```python
from build123d import *

# Parameters (mm, degrees)
SKETCH_W     = 12
SKETCH_H     = 12.3
PAD_DEPTH    = 2
SKETCH001_W  = 1.8
SKETCH001_H  = 2.7
POCKET_DEPTH = 0.2
PAD001_DEPTH = 13
CHAMFER_SIZE = 1


with BuildPart() as part:
    # Sketch → Pad (new body)
    with BuildSketch(Plane.XY):
        with Locations((6, 6.15)):
            Rectangle(SKETCH_W, SKETCH_H)
    extrude(amount=PAD_DEPTH)

    # Sketch001 (on Face5 of Pad) → Pocket (cut)
    with BuildSketch(Plane(origin=(0, 0, 0), x_dir=(1, 0, 0), z_dir=(0, 0, -1))):
        with Locations((6.2, -3.25)):
            Rectangle(SKETCH001_W, SKETCH001_H)
        with Locations((6.2, -9.05)):
            Rectangle(SKETCH001_W, SKETCH001_H)
    extrude(amount=-POCKET_DEPTH, mode=Mode.SUBTRACT)

    # Sketch002 (on Face1 of Pocket) → Pad001 (join)
    with BuildSketch(Plane.XZ):
        with BuildLine():
            ThreePointArc((11.16, 0.23875), (16.969381, -4.45007), (22.238211, 0.838915))
            Line((21.467655, 1.119375), (22.238211, 0.838915))
            ThreePointArc((12, 0), (17.23124, -3.647424), (21.467655, 1.119375))
            Line((12, 2), (12, 0))
            ThreePointArc((20.026412, 4.478132), (15.266374, 5.657977), (12, 2))
            Line((20.026412, 4.478132), (20.026412, 5.572296))
            ThreePointArc((20.026412, 5.572296), (14.583244, 6.292865), (11.16, 2))
            Line((11.16, 2), (11.16, 0.23875))
        make_face()
    extrude(amount=-PAD001_DEPTH)

    # Chamfer
    chamfer_edges = [part.edges().sort_by_distance(p)[0] for p in [
        (0, 6.15, 2),
    ]]
    chamfer(chamfer_edges, length=CHAMFER_SIZE)


solid = part.part
```
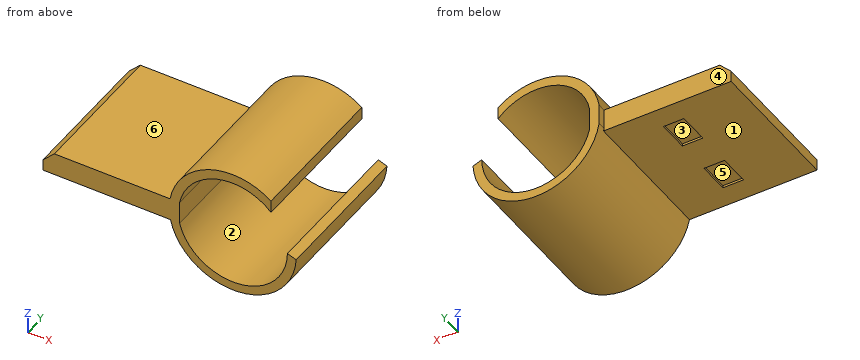
Could you check a few things on this model? Use its own coordinates, in mm. Face numbers are marked on the shaded views. A direction names the side the tool comes from. Give positions to 0.01 mm unless a question says otherwise; leave off trailing zeros. Write each loop counter-clockwise with the first axis right and the second up, starting at its lowest first coordinate (ties: lowest second). Pieces come first, ordered by that corner, then holes. Notation, with made-up numbers: (14, 7.5) - (63, 7.5) arc R17 ccw to (63, 34.5) - close; hole circle Ø5 at (15.25, -21.5). An arc over 180 degrees is marked (long way). One line per item, written item: value. Start each with the question number.
Item 1: Please list where these lines run through material, in increasing order: line 1 (Z direction, x = 10.25, y = 9.25); line 2 (X direction, y = 4.25, z = -3); line 3 (X direction, y = 10.5, z = -1.75). Write a range as from..to.
Item 2: Imagine slicing it at B-B, the plane z = 5.25. List the corners of the cut face in (x, y) for me, and give its area (3 significant figures).
Item 3: Imagine slicing it at C-C, the plane y = 12. List the corners of the cut face in (x, z) for me.
Item 4: Imagine slicing it at D-D, the plane x = 5.75. List the corners of the cut face in (y, z) for me, and give its area (3 significant figures).
Item 5: I'm going to push flat-ended pins straight in: pin 1 (3 mm diameter, centred on x = 6, y = 11, fed in from +Z); pin 2 (2 mm diameter, centred on x = 7, z = 1.5, fed in from +Y); pin 3 (1 mm diameter, centred on y = 9.5, z = -1.5, fed in from +X). Where does each tip first touch, or does it pass through?
Item 6: Imagine slicing it at A-A, the plane x = 17.75. List the corners of the cut face in (y, z) for me, and give its area (3 significant figures).
Item 7: Which directions (+Z, -Z, +X, -X, +Y, -Y) give clear straight access to the entire face, cutting with the end or side of a thin tool? Please do the marked faces 1, 2 and 3.
Item 8: If we mould it in two halves opening along Y, with no side actions, what happens to the marked faces 4, 5 and 6? For each: +Y half, -Y half, draft (parallel to the pull), parting line (faces both ways), or undercut.
Geometry says:
1. line 1: 0..2
1. line 2: 12.91..14.2, 19.13..20.43
1. line 3: 11.88..12.82, 20.52..21.45
2. outline: (12.92, 0) - (14.32, 0) - (14.32, 13) - (12.92, 13) - close; (19.01, 0) - (20.03, 0) - (20.03, 13) - (19.01, 13) - close
2. area: 31.4 mm^2
3. outline: (0, 0) - (11.2, 0) arc R5.58 ccw to (22.24, 0.84) - (21.47, 1.12) arc R4.8 cw to (12, 0) - (12, 2) arc R4.75 cw to (20.03, 4.48) - (20.03, 5.57) arc R5.58 ccw to (11.16, 2) - (1, 2) - (0, 1) - close
4. outline: (0, 0) - (1.9, 0) - (1.9, 0.2) - (4.6, 0.2) - (4.6, 0) - (7.7, 0) - (7.7, 0.2) - (10.4, 0.2) - (10.4, 0) - (12.3, 0) - (12.3, 2) - (0, 2) - close
4. area: 23.5 mm^2
5. pin 1: z = 2
5. pin 2: y = 12.3
5. pin 3: x = 21.83
6. outline: (0, -4.35) - (13, -4.35) - (13, -3.56) - (0, -3.56) - close; (0, 5.74) - (13, 5.74) - (13, 6.59) - (0, 6.59) - close
6. area: 21.3 mm^2
7. face 1: -Z, -X, +Y, -Y
7. face 2: +Y, -Y
7. face 3: -Z
8. face 4: +Y half
8. face 5: undercut
8. face 6: draft
